Geometry check sheet. Reference: the model listing, model coordinates, mm. A direction names the side the tool comes from. Give positions to 0.01 mm unless a question says otherwise; leave off trailing zeros. Loops run counter-clockwise (first coordinate to the right, second up) from the corner with the lowest first, then second, coordinate; pieces in that order, holes last.
```python
from build123d import *

# Parameters (mm, degrees)
F1_DEPTH = 19.05
F3_DEPTH = 17.2409580479
F5_DEPTH = 25.4
F6_W     = 23.5642232001
F6_H     = 34.1768339276
F7_DEPTH = 10.16


with BuildPart() as f1:
    # F0 (on Front) → F1 (new body, symmetric)
    with BuildSketch(Plane.XZ):
        Polygon((17.4721237272, 74.0977823734), (0, 74.0977823734), (0, 0), (55.0666376948, 0), (55.0666376948, 17.2399580479), (17.4721237272, 17.2399580479), align=None)
    extrude(amount=F1_DEPTH, both=True)

    # F2 (on face) → F3 (cut, through all)
    with BuildSketch(Plane.XY.offset(17.2399580479)):
        with BuildLine():
            ThreePointArc((55.0666376948, -0.3249626733), (51.4285906353, -11.785735895), (41.846567036, -19.05))
            Line((41.846567036, -19.05), (55.0666376948, -19.05))
            Line((55.0666376948, -19.05), (55.0666376948, -0.3249626733))
        make_face()
        with BuildLine():
            ThreePointArc((39.6085269749, 19.05), (50.7285952231, 12.0680027235), (55.0666376948, -0.3249626733))
            Line((55.0666376948, -0.3249626733), (55.0666376948, 19.05))
            Line((55.0666376948, 19.05), (39.6085269749, 19.05))
        make_face()
    extrude(amount=-F3_DEPTH, mode=Mode.SUBTRACT)

    # F4 (on face) → F5 (cut)
    with BuildSketch(Plane.YZ.offset(17.4721237272)):
        with BuildLine():
            Line((5.6702466682, 74.0977823734), (-5.6702466682, 74.0977823734))
            Line((-5.6702466682, 74.0977823734), (-5.6702466682, 38.6781468987))
            ThreePointArc((-5.6702466682, 38.6781468987), (0, 33.0079002306), (5.6702466682, 38.6781468987))
            Line((5.6702466682, 38.6781468987), (5.6702466682, 74.0977823734))
        make_face()
    extrude(amount=-F5_DEPTH, mode=Mode.SUBTRACT)

    # F6 (on face) → F7 (cut)
    with BuildSketch(Plane.XZ.offset(19.05)):
        with Locations((11.7821116, 11.8823200464)):
            Rectangle(F6_W, F6_H)
    extrude(amount=-F7_DEPTH, mode=Mode.SUBTRACT)


solid = f1.part
```
1) Mould release check, pull along Y, two halves, no side actions. Record for faces 6 (the flat face through (0, 0, 29)), 7 (the flat face through (9, 5.67, 56)), 8 (the flat face through (11, 19.05, 29)), 9 (the flat face through (12, -8.89, 15)): +Y half, -Y half, draft (parallel to the pull), parting line (faces both ways), or undercut.
2) Sectioned sample at D-D on x = 25. Enter the section's corners in (y, z), plus the area to 3 significant figures.
3) Sectioned sample at C-C on y = -13. Enter the section's corners in (x, z), plus the area to 3 significant figures.
4) Depth check by flat-ended pin: P1, Ø3, axis at y = -14.5, z = 10.5, coming from the -X side; P2, Ø2, axis at x = 13, z = 17, coming from the -Y side; P3, Ø1.5, axis at y = 12.5, z = 43.5, coming from the +X side. Enter the tip coordinate at first touch or a pass-through.
5) Sectioned sample at A-A on z = 41. Enter the section's corners in (x, y).
6) Sectioned sample at B-B on z = 16. Enter the section's corners in (x, y), plus the area to 3 significant figures.
7) Scan lines: line 1 along X through (y, z) = (0.5, 11.5); line 2 along Z through (x, y) = (26, -8); line 3 along Y through (x, z) = (13, 33.5). Record each from-to range of solid material in increasing order.
8) Tool access check on faces 1 (the flat face through (33, -19.05, 9)), 2 (the flat face through (9, -14, 28.971)), 3 (the flat face through (23.564, -14, 8)), 4 (the flat face through (17.472, 8, 45)), 5 (the flat face through (9, -5.67, 57)). Record the directions out of +Z, -Z, +X, -X, +Y, -Y that give a thin tool (end or side, any length) a straight path to the whole face; none if there is none.
Determined:
1. face 6: draft
1. face 7: undercut
1. face 8: +Y half
1. face 9: -Y half
2. outline: (-19.05, 0) - (19.05, 0) - (19.05, 17.24) - (-19.05, 17.24) - close
2. area: 657 mm2
3. outline: (0, 28.97) - (17.47, 28.97) - (17.47, 74.1) - (0, 74.1) - close; (23.56, 0) - (50.5, 0) - (50.5, 17.24) - (23.56, 17.24) - close
3. area: 1,250 mm2
4. P1: stops at x = 23.56
4. P2: stops at y = -8.89
4. P3: stops at x = 17.47
5. outline: (0, -19.05) - (17.47, -19.05) - (17.47, -5.67) - (0, -5.67) - close; (0, 5.67) - (17.47, 5.67) - (17.47, 19.05) - (0, 19.05) - close
6. outline: (0, -8.89) - (23.56, -8.89) - (23.56, -19.05) - (41.85, -19.05) arc R19.87 ccw to (39.61, 19.05) - (0, 19.05) - close
6. area: 1,720 mm2
7. line 1: x = 0 to 55.05
7. line 2: z = 0 to 17.24
7. line 3: y = -19.05 to -2.31, 2.31 to 19.05
8. face 1: +Z, -Z, +X, -X, -Y
8. face 2: -Z, +X, -X, -Y
8. face 3: +Z, -Z, -X, -Y
8. face 4: +Z, +X, +Y, -Y
8. face 5: +Z, +X, -X
